Input: part model. Units: mm. Frame: model coordinates. Face numbers are marked on the shaded views. A direction names the side the tool comes from. Round coordinates to 2 decimals unless told otherwise and drop trailing zeros. Loops run counter-clockwise (first coordinate to the right, second up) from the corner with the lowest first, then second, coordinate; pieces in that order, holes last. Notation, with made-up numbers: (-22.5, 45) - (11.5, 45) arc R25 cw to (11.5, 60) - close; hole circle Ø1 at (58.5, 80.5). An arc over 180 degrees is marked (long way). Write each question's results on one line, items separated by ' | '.
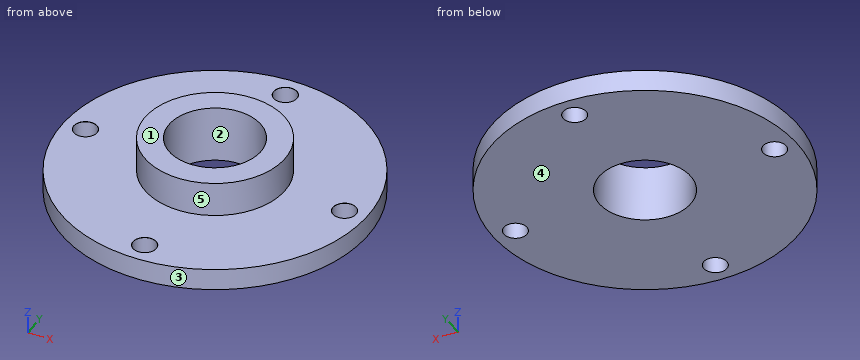
from build123d import *

# Parameters (mm, degrees)
SKETCH1_R                      = 35
SKETCH1_R_2                    = 10.5
BOSS_EXTRUDE1_DEPTH            = 5
M5_CLEARANCE_HOLE1_D           = 5.3
M5_CLEARANCE_HOLE1_CSINK_D     = 5.35
M5_CLEARANCE_HOLE1_CSINK_ANGLE = 90
CIRPATTERN1_COUNT              = 4
SKETCH5_R                      = 16
SKETCH5_R_2                    = 10.5
BOSS_EXTRUDE2_DEPTH            = 8


with BuildPart() as part:
    # Sketch1 → Boss-Extrude1 (new body)
    with BuildSketch(Plane.XY):
        Circle(SKETCH1_R)
        Circle(SKETCH1_R_2, mode=Mode.SUBTRACT)
    extrude(amount=BOSS_EXTRUDE1_DEPTH)

    # M5 Clearance Hole1 (through all)
    with Locations(Plane.XY.offset(5)):
        with Locations((0, 30)):
            m5_clearance_hole1 = CounterSinkHole(M5_CLEARANCE_HOLE1_D / 2, M5_CLEARANCE_HOLE1_CSINK_D / 2, counter_sink_angle=M5_CLEARANCE_HOLE1_CSINK_ANGLE)

    # CirPattern1: M5 Clearance Hole1 ×4 about axis
    cirpattern1_axis = Axis((0, 0, 0), (0, 0, 1))
    for i in range(1, CIRPATTERN1_COUNT):
        add(m5_clearance_hole1.rotate(cirpattern1_axis, i * 360 / CIRPATTERN1_COUNT), mode=Mode.SUBTRACT)

    # Sketch5 → Boss-Extrude2 (add)
    with BuildSketch(Plane.XY.offset(5)):
        Circle(SKETCH5_R)
        Circle(SKETCH5_R_2, mode=Mode.SUBTRACT)
    extrude(amount=BOSS_EXTRUDE2_DEPTH)


solid = part.part
1. Section query D-D, the plane y = 30. Output: boundary loops of the cut face in (x, z) (3 decimals), plus the area to 3 significant figures.
Answer:
outline: (-18.028, 0) - (-2.65, 0) - (-2.65, 4.975) - (-2.675, 5) - (-18.028, 5) - close; (2.65, 0) - (18.028, 0) - (18.028, 5) - (2.675, 5) - (2.65, 4.975) - close | area: 154 mm^2
2. Line query: line 1 (Y direction, x = 0, z = 3.6); line 2 (Y direction, x = 0, z = 5.5); line 3 (Z direction, x = -19, y = 2). Output: solid intervals per line, ascending. Write a range as [from, to].
Answer:
line 1: [-35, -32.65], [-27.35, -10.5], [10.5, 27.35], [32.65, 35] | line 2: [-16, -10.5], [10.5, 16] | line 3: [0, 5]
3. Section query C-C, the plane z = 2. Output: boundary loops of the cut face in (x, y).
Answer:
outline: circle Ø70 at (0, 0); hole circle Ø5.3 at (-30, 0); hole circle Ø21 at (0, 0); hole circle Ø5.3 at (0, -30); hole circle Ø5.3 at (0, 30); hole circle Ø5.3 at (30, 0)
4. Contact query for flat-ended pins moving along their axis: pin 1 (1 mm diameter, centred on x = -17.5, y = 19, fed in from +Z); pin 2 (5 mm diameter, centred on x = -30, y = 0, fed in from -Z); pin 3 (4 mm diameter, centred on x = 13, z = 2, fed in from -Y); pin 4 (5 mm diameter, centred on x = -3.5, z = 3, fed in from +Y). Output: stop coordinate, or through.
Answer:
pin 1: z = 5 | pin 2: through | pin 3: y = -33.23 | pin 4: y = 34.99
5. Set-up query: the marked faces 4 and 5. Return all of +Z, -Z, +X, -X, +Y, -Y with unobstructed straight access to the full face (end or side cutting, diameter ignored); none if empty.
Answer:
face 4: -Z, +X, -X, +Y, -Y | face 5: +Z
6. Mould query, pull axis X, two halves, no side actions, for the marked faces 1, 2 and 3. Classes: pulls with the +X half, pulls with the -X half, needs draft (parallel to the pull), parting line crosses it, or undercut.
Answer:
face 1: needs draft | face 2: undercut | face 3: parting line crosses it
7. Section query A-A, the plane x = 0. Output: boundary loops of the cut face in (y, z) (3 decimals).
Answer:
outline: (-35, 0) - (-32.65, 0) - (-32.65, 4.975) - (-32.675, 5) - (-35, 5) - close; (-27.35, 0) - (-10.5, 0) - (-10.5, 13) - (-16, 13) - (-16, 5) - (-27.325, 5) - (-27.35, 4.975) - close; (10.5, 0) - (27.35, 0) - (27.35, 4.975) - (27.325, 5) - (16, 5) - (16, 13) - (10.5, 13) - close; (32.65, 0) - (35, 0) - (35, 5) - (32.675, 5) - (32.65, 4.975) - close
